Design review of the part built by this model. Coordinates are the model's own, in mm. Coordinates: 2 decimals unless noted, no trailing zeros. Loops run counter-clockwise (first coordinate to the right, second up) from the corner with the lowest first, then second, coordinate; pieces in that order, holes last. Notation, with made-up numbers: M -6,35.5 L 11,35.5 A31 cw 11,60.5 Z; hole C 17.5,52 d2. An arc over 180 degrees is marked long. Answer as CSV lines item,"result". Start each with the question number.
from build123d import *

# Parameters (mm, degrees)
ESQUISSE1_R             = 4
BOSS_EXTRU_1_DEPTH      = 10
ENL_V_MAT_EXTRU_1_DEPTH = 607.65970692


with BuildPart() as part:
    # Esquisse1 → Boss.-Extru.1 (new body)
    with BuildSketch(Plane.XY):
        with BuildLine():
            Line((-452, -400), (452, -400))
            ThreePointArc((452, -400), (454.828427125, -398.828427125), (456, -396))
            Line((456, -396), (456, 396))
            ThreePointArc((456, 396), (454.828427125, 398.828427125), (452, 400))
            Line((452, 400), (-452, 400))
            ThreePointArc((-452, 400), (-454.828427125, 398.828427125), (-456, 396))
            Line((-456, 396), (-456, -396))
            ThreePointArc((-456, -396), (-454.828427125, -398.828427125), (-452, -400))
        make_face()
        with Locations((436, 380)):
            Circle(ESQUISSE1_R, mode=Mode.SUBTRACT)
        with Locations((435.5, -140)):
            Circle(ESQUISSE1_R, mode=Mode.SUBTRACT)
        with Locations((435.5, 141)):
            Circle(ESQUISSE1_R, mode=Mode.SUBTRACT)
        with Locations(Location((-435.5, -140, 0), (0, 0, 180))):
            Circle(ESQUISSE1_R, mode=Mode.SUBTRACT)
        with Locations(Location((-436, 380, 0), (0, 0, 180))):
            Circle(ESQUISSE1_R, mode=Mode.SUBTRACT)
        with Locations(Location((-435.5, 141, 0), (0, 0, 180))):
            Circle(ESQUISSE1_R, mode=Mode.SUBTRACT)
        with Locations(Location((436, -380, 0), (0, 0, 180))):
            Circle(ESQUISSE1_R, mode=Mode.SUBTRACT)
        with Locations(Location((436, -340, 0), (0, 0, 180))):
            Circle(ESQUISSE1_R, mode=Mode.SUBTRACT)
        with Locations((-436, -340)):
            Circle(ESQUISSE1_R, mode=Mode.SUBTRACT)
        with Locations((-436, -380)):
            Circle(ESQUISSE1_R, mode=Mode.SUBTRACT)
        with Locations(Location((218, -380, 0), (0, 0, 180))):
            Circle(ESQUISSE1_R, mode=Mode.SUBTRACT)
        with Locations(Location((0, -380, 0), (0, 0, 180))):
            Circle(ESQUISSE1_R, mode=Mode.SUBTRACT)
        with Locations(Location((-218, -380, 0), (0, 0, 180))):
            Circle(ESQUISSE1_R, mode=Mode.SUBTRACT)
        with Locations((-218, 380)):
            Circle(ESQUISSE1_R, mode=Mode.SUBTRACT)
        with Locations((0, 380)):
            Circle(ESQUISSE1_R, mode=Mode.SUBTRACT)
        with Locations((218, 380)):
            Circle(ESQUISSE1_R, mode=Mode.SUBTRACT)
    extrude(amount=BOSS_EXTRU_1_DEPTH)

    # Esquisse2 → Enlèv. mat.-Extru.1 (cut, through all)
    with BuildSketch(Plane.XY.offset(10)):
        with BuildLine():
            Line((-125, -200), (125, -200))
            ThreePointArc((125, -200), (142.67766953, -192.67766953), (150, -175))
            Line((150, -175), (150, 175))
            ThreePointArc((150, 175), (142.67766953, 192.67766953), (125, 200))
            Line((125, 200), (-125, 200))
            ThreePointArc((-125, 200), (-142.67766953, 192.67766953), (-150, 175))
            Line((-150, 175), (-150, -175))
            ThreePointArc((-150, -175), (-142.67766953, -192.67766953), (-125, -200))
        make_face()
    extrude(amount=-ENL_V_MAT_EXTRU_1_DEPTH, mode=Mode.SUBTRACT)


solid = part.part
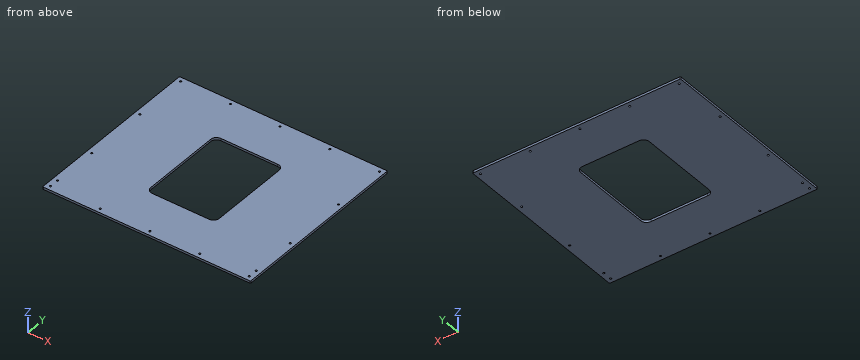
Item 1: Add section B-B (x = 83). Give the boundary of the cut face in (y, z), plus the area to 3 significant figures.
Item 2: Add section A-A (z = 5.5). Give the number of separate pieces and of enclosed holes in the cut face, plus the area to 3 significant figures.
Item 3: For line 1 along Y through (x, z) = (-218, 2.75); line 2 along X through (y, z) = (380, 6.75); line 3 along X through (y, z) = (-340, 6.5), list the stretches that pass through material, from the lowest coordinate up. Write a range as from..to.
Response:
1,outline,"M -400,0 L -200,0 L -200,10 L -400,10 Z; M 200,0 L 400,0 L 400,10 L 200,10 Z"
1,area,"4,000 mm²"
2,separate pieces,"1"
2,enclosed holes,"17"
2,area,"609,000 mm²"
3,line 1,"-400..-384, -376..376, 384..400"
3,line 2,"-456..-440, -432..-222, -214..-4, 4..214, 222..432, 440..456"
3,line 3,"-456..-440, -432..432, 440..456"
